```python
from build123d import *

# Parameters (mm, degrees)
EXTRUDE_1_DEPTH     = 10
SKETCH_2_R          = 4.2
CUT_EXTRUDE_1_DEPTH = 40.634142812
FILLET_1_R          = 5
FILLET_2_R          = 5
FILLET_3_R          = 5


with BuildPart() as part:
    # 草图1 → 凸台-拉伸1 (new body)
    with BuildSketch(Plane(origin=(0, 0, 0), x_dir=(1, 0, 0), z_dir=(0, 1, 0))):
        with BuildLine():
            ThreePointArc((-21.701095489, -19.186348515), (3.298904511, -25.885078326), (28.298904511, -19.186348515))
            ThreePointArc((28.298904511, -19.186348515), (21.6001747, 5.813651485), (3.298904511, 24.114921674))
            ThreePointArc((3.298904511, 24.114921674), (-15.002365678, 5.813651485), (-21.701095489, -19.186348515))
        make_face()
    extrude(amount=EXTRUDE_1_DEPTH)

    # 草图2 → 切除-拉伸1 (cut, through all)
    with BuildSketch(Plane(origin=(0, 10, 0), x_dir=(1, 0, 0), z_dir=(0, 1, 0))):
        with Locations(Location((3.298904511, 9.114921674, 0), (0, 0, 270))):
            Circle(SKETCH_2_R)
    extrude(amount=-CUT_EXTRUDE_1_DEPTH, mode=Mode.SUBTRACT)

    # 圆角1
    fillet_1_edges = [part.edges().sort_by_distance(p)[0] for p in [
        (3.298904511, 5, -24.114921674),
    ]]
    fillet(fillet_1_edges, radius=FILLET_1_R)

    # 圆角2
    fillet_2_edges = [part.edges().sort_by_distance(p)[0] for p in [
        (-21.701095489, 5, 19.186348515),
    ]]
    fillet(fillet_2_edges, radius=FILLET_2_R)

    # 圆角3
    fillet_3_edges = [part.edges().sort_by_distance(p)[0] for p in [
        (28.298904511, 5, 19.186348515),
    ]]
    fillet(fillet_3_edges, radius=FILLET_3_R)


solid = part.part
```
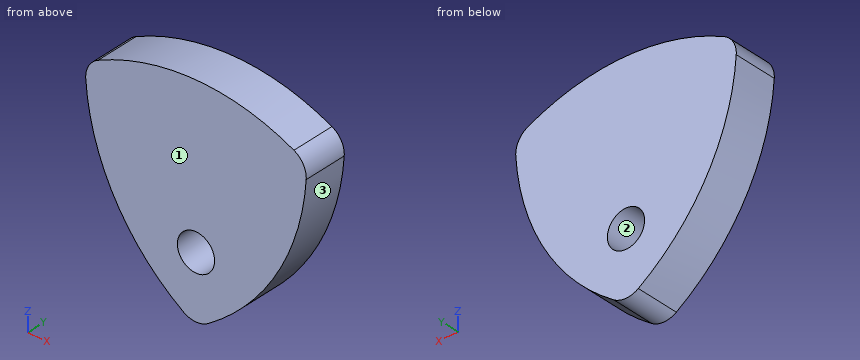
Read the model definition and answer for the solid it produces. Units are mm, in the model's axes. Face numbers are marked on the shaded views. Coordinates: 2 decimals unless noted, no trailing zeros. Write each loop counter-clockwise with the first axis right and the second up, starting at its lowest first coordinate (ties: lowest second). Pieces come first, ordered by that corner, then holes. Notation, with made-up numbers: (3, 32) -> (17, 32) arc R22 ccw to (17, 40) -> close; hole circle Ø4 at (-6.75, 40). An arc over 180 degrees is marked (long way). Answer as a JSON object with one key per item and string values.
Q1. The part is cut by section B-B on z = 21.5. Give the vertices of the cut face in (x, y), then the cut area to 3 significant figures.
The answers:
{"outline": "(-17.18, 0) -> (23.78, 0) -> (23.78, 10) -> (-17.18, 10) -> close", "area": "410 mm2"}
Q2. Flat-ended cylindrical pins translate along their axes: pin 1 Ø5 at (x, y) = (17.5, 6) entering from +Z; pin 2 Ø1.5 at (y, z) = (5, -7.5) entering from -X; pin 3 Ø1.5 at (y, z) = (4, 5.5) entering from -X. Find the tip coordinate at first contact, or state that the pin passes through.
The answers:
{"pin 1": "stops at z = 24.5", "pin 2": "stops at x = -14.45", "pin 3": "stops at x = -20"}
Q3. Determine the mould class of the marked faces 1, 2 and 3 for opening direction Z: pulls with the +Z half, pulls with the -Z half, needs draft (parallel to the pull), parting line crosses it, or undercut.
The answers:
{"face 1": "needs draft", "face 2": "undercut", "face 3": "pulls with the -Z half"}
Q4. Consider line 1 (Z direction, x = -0.5, y = 5.75); line 2 (X direction, y = 6.75, z = -12); line 3 (X direction, y = 1.75, z = -11). Determine where each line is inside the solid, lowest interval first. Write a range as [from, to].
The answers:
{"line 1": "z = [-21.69, -10.91], [-7.32, 25.74]", "line 2": "x = [-10.78, 0.25], [6.35, 17.38]", "line 3": "x = [-11.56, -0.45], [7.05, 18.16]"}
Q5. The part is cut by section A-A on x = 15. Give the vertices of the cut face in (y, z).
The answers:
{"outline": "(0, -14.77) -> (10, -14.77) -> (10, 24.5) -> (0, 24.5) -> close"}
